Geometry: see drawing. Coordinates: mm, zero at the bounding-box minimum. Round coordinates to 2 decimals unless told otherwise and drop trailing zeros. Write each loop counter-clockwise with the first axis right and the second up, starting at its lowest first coordinate (ties: lowest second). Pieces come first, ordered by that corner, then holes. Notation, with made-up numbers: M -17,-24.5 L 36,-24.5 A20 ccw 36,2.5 Z; hole C 70,-34.75 d6. An arc over 180 degrees is marked long. Use a Markdown table: item, result.
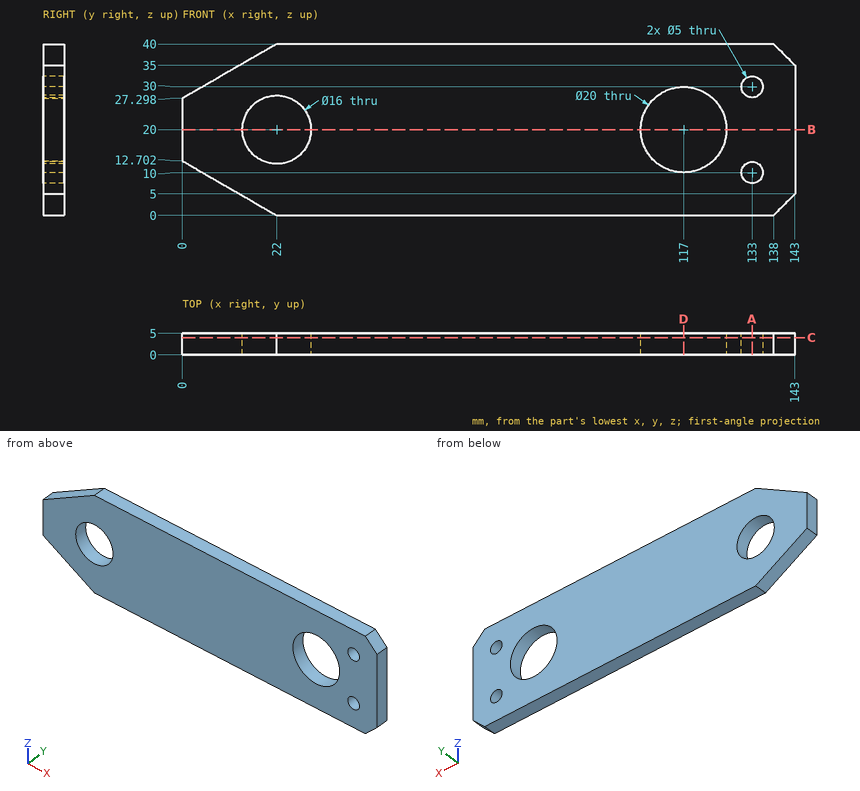
Q1. Line query: L1, parallel to Z at x = 133, y = 1; L2, parallel to X at y = 2.75, z = 25.5; L3, parallel to Z at x = 125.5, y = 0.7. Output: solid intervals per line, ascending.
Results are:
| item | result |
|---|---|
| L1 | 0 to 7.5, 12.5 to 27.5, 32.5 to 40 |
| L2 | 0 to 16.19, 27.81 to 108.65, 125.35 to 143 |
| L3 | 0 to 14.73, 25.27 to 40 |
Q2. Section D-D on x = 117. Return loops of the section in (y, z).
Results are:
| item | result |
|---|---|
| outline | M 0,0 L 5,0 L 5,10 L 0,10 Z; M 0,30 L 5,30 L 5,40 L 0,40 Z |
Q3. Section C-C on y = 4. Return loops of the section in (x, z), plus the area to 3 significant figures.
Results are:
| item | result |
|---|---|
| outline | M 0,12.7 L 22,0 L 138,0 L 143,5 L 143,35 L 138,40 L 22,40 L 0,27.3 Z; hole C 22,20 d16; hole C 117,20 d20; hole C 133,10 d5; hole C 133,30 d5 |
| area | 4,860 mm^2 |
Q4. Section A-A on x = 133. Return loops of the section in (y, z), plus the area to 3 significant figures.
Results are:
| item | result |
|---|---|
| outline | M 0,0 L 5,0 L 5,7.5 L 0,7.5 Z; M 0,12.5 L 5,12.5 L 5,27.5 L 0,27.5 Z; M 0,32.5 L 5,32.5 L 5,40 L 0,40 Z |
| area | 150 mm^2 |
Q5. Section B-B on z = 20. Return loops of the section in (x, y), plus the area to 3 significant figures.
Results are:
| item | result |
|---|---|
| outline | M 0,0 L 14,0 L 14,5 L 0,5 Z; M 30,0 L 107,0 L 107,5 L 30,5 Z; M 127,0 L 143,0 L 143,5 L 127,5 Z |
| area | 535 mm^2 |
